Geometry: see drawing. Coordinates: mm, zero at the bounding-box minimum. Give positions to 0.01 mm unless a question says otherwise; leave off trailing zeros. Loops run counter-clockwise (first coordinate to the right, second up) from the corner with the lowest first, then second, coordinate; pieces in that order, holes last. Notation, with made-up numbers: (0.5, 0.25) -> (34.5, 0.25) arc R31 ccw to (34.5, 36.25) -> close; hole circle Ø11 at (21, -13). An arc over 180 degrees is marked (long way). Answer in a Markdown table with one row per item. Add a question column.
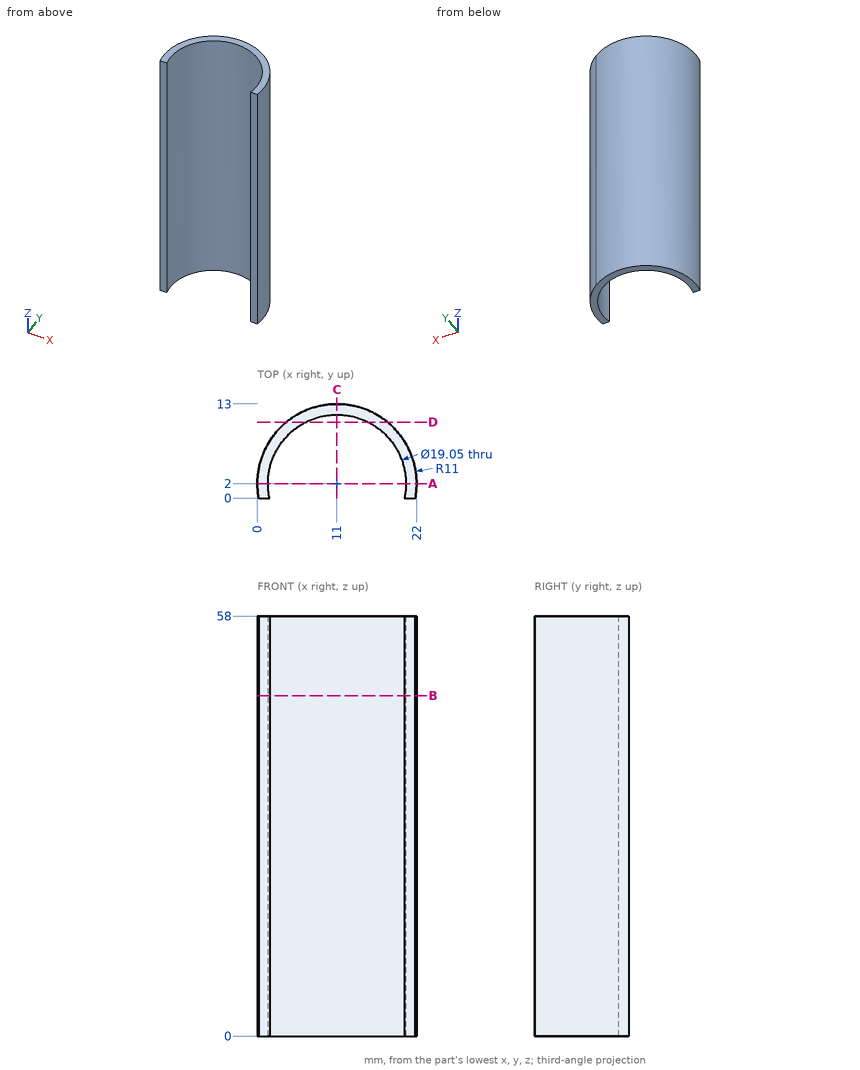
1) Section B-B on z = 47. Output: boundary loops of the cut face in (x, y) (3 decimals).
2) Pin query (flat end, axial travel): pin 1 (6 mm diameter, centred on x = 3, z = 32, fed in from +Y); pin 2 (4 mm diameter, centred on y = 10, z = 31.5, fed in from +X); pin 3 (5 mm diameter, centred on x = 15.5, y = 3, fed in from -Z); pin 4 (6 mm diameter, centred on y = 11, z = 12, fed in from -X). Return the tip coordinate at first contact, or that it passes through.
3) Section C-C on x = 11. Output: boundary loops of the cut face in (y, z) (3 decimals).
4) Material intervals for line 1 along X through (y, z) = (2, 20) (3 decimals); line 2 along Y through (x, z) = (11, 38) (3 decimals); line 3 along X through (y, z) = (8.25, 42), sorted ascending.
5) Section D-D on y = 10.5. Output: boundary loops of the cut face in (x, z), and give its area (3 significant figures).
6) Section A-A on y = 2. Output: boundary loops of the cut face in (x, z) (3 decimals).
Working result:
| question | item | result |
|---|---|---|
| 1 | outline | (0.183, 0) -> (1.687, 0) arc R9.525 cw (long way) to (20.313, 0) -> (21.817, 0) arc R11 ccw to (20.666, 7.25) arc R11 ccw to (17.176, 11.103) arc R11 ccw to start |
| 2 | pin 1 | stops at y = 11.8 |
| 2 | pin 2 | stops at x = 20.22 |
| 2 | pin 3 | passes through |
| 2 | pin 4 | stops at x = 1.78 |
| 3 | outline | (11.525, 0) -> (13, 0) -> (13, 58) -> (11.525, 58) -> close |
| 4 | line 1 | x = 0 to 1.475, 20.525 to 22 |
| 4 | line 2 | y = 11.525 to 13 |
| 4 | line 3 | x = 1.95 to 3.81, 18.19 to 20.05 |
| 5 | outline | (4.02, 0) -> (6.7, 0) -> (6.7, 58) -> (4.02, 58) -> close; (15.3, 0) -> (17.98, 0) -> (17.98, 58) -> (15.3, 58) -> close |
| 5 | area | 311 mm2 |
| 6 | outline | (0, 0) -> (1.475, 0) -> (1.475, 58) -> (0, 58) -> close; (20.525, 0) -> (22, 0) -> (22, 58) -> (20.525, 58) -> close |
